Read the model definition and answer for the solid it produces. Units are mm, in the model's axes. A direction names the side the tool comes from. Coordinates: 2 decimals unless noted, no trailing zeros. Loops run counter-clockwise (first coordinate to the right, second up) from the corner with the lowest first, then second, coordinate; pieces in that order, holes last. Notation, with made-up numbers: M 1,44 L 59,44 A18 cw 59,48 Z; hole C 32,-20 d5. An arc over 180 degrees is marked long. Use one line per item in the form item = value. Start each with the question number.
1. The part is cut by section B-B (y = -59). Give the vertices of the cut face in (x, z), plus the area to 3 significant figures.
2. For a pull along Y with two mould halves and no side action, classify faces 1 (the flat face through (12, 0, -37)), 2 (the cylindrical face through (-6.883, -21.648, -30.995)), 3 (the conical face through (12.846, -44.925, 30.983)) as released by +Y, released by -Y, zero draft, split by the parting line, or undercut.
3. Find the intervals of material crossed by probe 1 along X at (y, z) = (-15.5, 0) (3 decimals); probe 2 along X at (y, z) = (-100.5, 0), in increasing order. Write a range as [from, to].
4. The part is cut by section A-A (y = -86). Give the vertices of the cut face in (x, z) (1 decimal).
5. A tool of negligible diameter and unlimited length cuts with its end or side. For faces 4 (the cylindrical face through (-13.83, -100.87, 43.91)), 5 (the cylindrical face through (-6.194, -19.343, -27.895)), 6 (the conical face through (14.15, -45.594, 34.128)), from which of +Z, -Z, +X, -X, +Y, -Y can it reach the whole face along a straight path? Write none if from no direction.
6. Flat-ended cylindrical pins translate along their axes: pin 1 (3 mm diameter, centred on y = -89.5, z = 24.5, fed in from +X); pin 2 (2 mm diameter, centred on x = 8, y = -82.5, fed in from +Z); pin 3 (4 mm diameter, centred on y = -91, z = 1.5, fed in from -X). Find the tip coordinate at first contact, or state that the pin passes through.
from build123d import *

# Parameters (mm, degrees)
F0_R     = 57.15
F1_DEPTH = 5.08
F2_R     = 31.75
F3_DEPTH = 25.4
F4_R     = 28.575
F5_DEPTH = 30.481
F8_W     = 38.1
F8_H     = 3.175
F10_R    = 9.525
F11_R    = 9.525


with BuildPart() as f1:
    # F0 (on Front) → F1 (new body)
    with BuildSketch(Plane.XZ):
        Circle(F0_R)
    extrude(amount=F1_DEPTH)

    # F2 (on face) → F3 (join)
    with BuildSketch(Plane.XZ.offset(5.08)):
        Circle(F2_R)
    extrude(amount=F3_DEPTH)

    # F4 (on face) → F5 (cut, through all)
    with BuildSketch(Plane.XZ.offset(30.48)):
        Circle(F4_R)
    extrude(amount=-F5_DEPTH, mode=Mode.SUBTRACT)

    # F6 (on Right) → F7 (revolve)
    with BuildSketch(Plane.YZ):
        Polygon((-81.28, 46.0375), (-30.48, 28.575), (-30.48, 31.75), (-81.28, 49.2125), align=None)
    revolve(axis=Axis((0, -18.848058, 0), (0, -1, 0)))

    # F8 (on Right) → F9 (revolve)
    with BuildSketch(Plane.YZ):
        with Locations((-100.33, 47.625)):
            Rectangle(F8_W, F8_H)
    revolve(axis=Axis((0, -63.416593, 0), (0, -1, 0)))

    # F10
    f10_edges = [f1.edges().sort_by_distance(p)[0] for p in [
        (-31.75, -5.08, 0),
        (-22.45064, -30.48, -22.45064),
        (0, -81.28, -49.2125),
    ]]
    fillet(f10_edges, radius=F10_R)

    # F11
    f11_edges = [f1.edges().sort_by_distance(p)[0] for p in [
        (-28.575, 0, 0),
        (-20.205576, -30.48, -20.205576),
        (0, -81.28, -46.0375),
    ]]
    fillet(f11_edges, radius=F11_R)


solid = f1.part
Computed values:
q1.outline = C 0,0 d83.11; hole C 0,0 d76.76
q1.area = 797 mm²
q2.face_1 = released by +Y
q2.face_2 = undercut
q2.face_3 = released by -Y
q3.probe_1 = [-31.75, -28.575], [28.575, 31.75]
q3.probe_2 = [-49.21, -46.04], [46.04, 49.21]
q4.outline = C 0,0 d98.4; hole C 0,0 d92.1
q5.face_4 = -Y
q5.face_5 = +Y, -Y
q5.face_6 = none
q6.pin_1 = 43.51
q6.pin_2 = 48.71
q6.pin_3 = -49.21
